Part print with two shaded views. Sizes in mm from the minimum x, y, z corner. A direction names the side the tool comes from. Coordinates: 2 decimals unless noted, no trailing zeros. Order: outer loops, then holes, each group sorted by start corner. A loop starts at its lowest first (then second) coordinate and runs counter-clockwise, first axis right, second up. Notation, with made-up numbers: (10, 65) - (21, 65) arc R35 cw to (21, 104) - close; hole circle Ø10 at (12, 18). An arc over 180 degrees is marked (long way). Return JSON: item names as keys, results as strings.
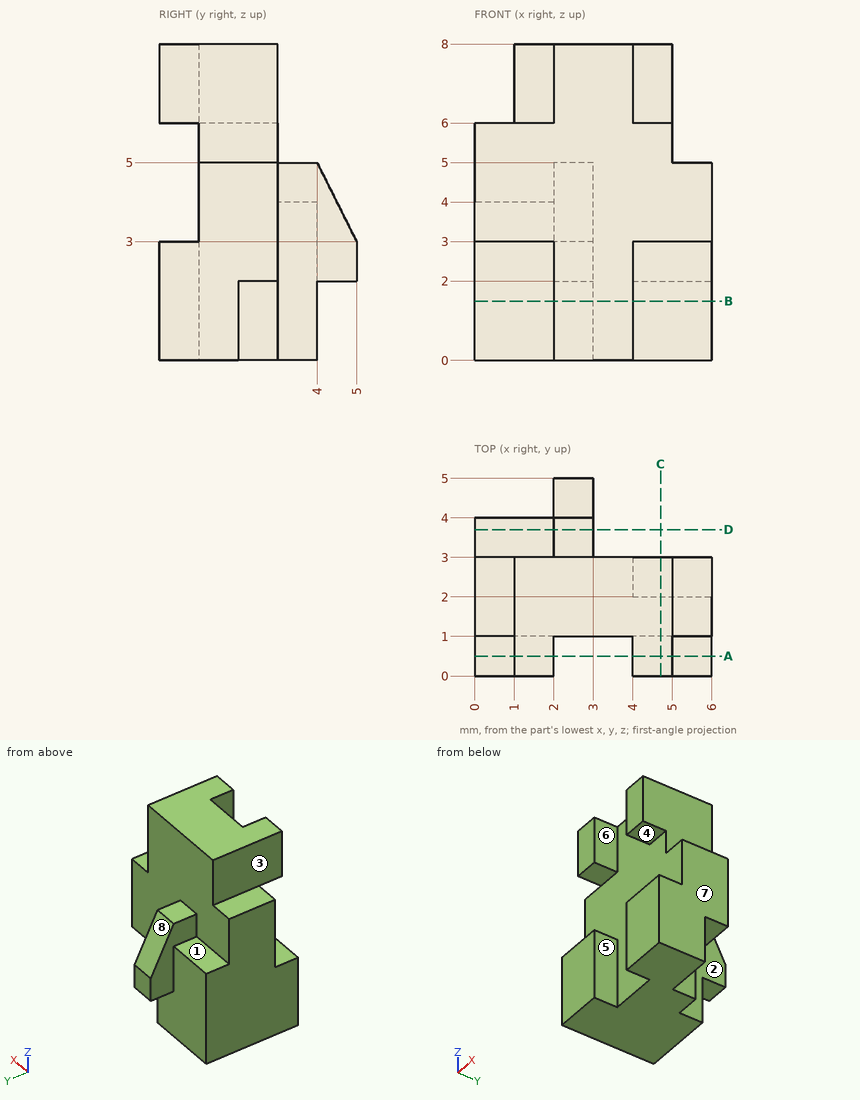
Item 1: Band-saw the part on C-C, the plane x = 4.7. List the corners of the cut face in (y, z).
Findings below:
{"outline": "(0, 0) - (2, 0) - (2, 2) - (3, 2) - (3, 8) - (0, 8) - (0, 6) - (1, 6) - (1, 3) - (0, 3) - close"}
Item 2: Which spindle directions (+Z, -Z, +X, -X, +Y, -Y) get a long thin tool onto all of the face, cutting with end or side? Do the marked faces 1, 2, 3, 4 and 5. Say none if no direction does.
Findings below:
{"face 1": "+Z, -X, +Y", "face 2": "+Z, -Z, +X, +Y", "face 3": "+Z, -X, +Y, -Y", "face 4": "+X, -X, -Y", "face 5": "+Z, -Z, -Y"}
Item 3: Mould opens along X. For the marked faces 6, 7 and 8 say: released by +X, released by -X, zero draft, split by the parting line, or undercut.
Findings below:
{"face 6": "undercut", "face 7": "released by +X", "face 8": "zero draft"}
Item 4: Band-saw the part on B-B, the plane z = 1.5. List the corners of the cut face in (x, y).
Findings below:
{"outline": "(0, 0) - (2, 0) - (2, 1) - (4, 1) - (4, 0) - (6, 0) - (6, 2) - (4, 2) - (4, 3) - (3, 3) - (3, 4) - (0, 4) - close"}
Item 5: Drop flat-ended pins along their axis: P1, Ø0.8, axis at y = 2.5, z = 1.5, coming from the +X side; P2, Ø1, axis at y = 2, z = 7, coming from the -X side; P3, Ø0.5, axis at y = 0.5, z = 7, coming from the +X side. Give the stop position or say it passes through.
Findings below:
{"P1": "stops at x = 4", "P2": "stops at x = 1", "P3": "stops at x = 5"}
Item 6: Band-saw the part on D-D, the plane y = 3.7. List the corners of the cut face in (x, z), then the cut area to 3 significant figures.
Findings below:
{"outline": "(0, 0) - (3, 0) - (3, 5) - (2, 5) - (2, 4) - (0, 4) - close", "area": "13.0 mm²"}
Item 7: Band-saw the part on A-A, the plane y = 0.5. List the corners of the cut face in (x, z).
Findings below:
{"outline": "(0, 0) - (2, 0) - (2, 3) - (0, 3) - close; (1, 6) - (2, 6) - (2, 8) - (1, 8) - close; (4, 0) - (6, 0) - (6, 3) - (4, 3) - close; (4, 6) - (5, 6) - (5, 8) - (4, 8) - close"}
Item 8: Wall check: L1, parallel to X at y = 0.45, z = 2; L2, parallel to X at y = 0.9, z = 6.25; L3, parallel to Z at x = 1.45, y = 3.4. Give the ranges that are in metal, low to high. Write a range as [from, to].
Findings below:
{"L1": "x = [0, 2], [4, 6]", "L2": "x = [1, 2], [4, 5]", "L3": "z = [0, 4]"}
